Drawing for the job (mm, zero at the part's lowest x, y, z). A direction names the side the tool comes from. Give positions to 0.01 mm unless a question says otherwise; leave off trailing zeros. Order: outer loops, then holes, each group sorted by start corner. A loop starts at its lowest first (then second) coordinate and runs counter-clockwise, first axis right, second up. Notation, with made-up numbers: (70, 22.25) - (94, 22.25) arc R15 cw to (94, 47.25) - close; hole circle Ø6 at (35.25, 39.5). An arc over 180 degrees is marked (long way). Use a Markdown table: item, result. Add a question column.
(1) Flat gauge pins, fed straight in: pin 1 (10 mm diameter, centred on x = 56.5, z = 29, fed in from +Y); pin 2 (1.5 mm diameter, centred on x = 40, y = 25.5, fed in from -Z); pin 3 (1.1 mm diameter, centred on x = 49, y = 56, fed in from +Z); pin 4 (1 mm diameter, centred on x = 8, y = 47, fed in from +Z). Where does each tip first touch, or does it go through?
(2) Slice it at B-B (x = 39). Write the cut outline in (y, z).
(3) Mould opens along Y. For the marked faces 3, 4 and 5 say: +Y half, -Y half, draft (parallel to the pull), parting line (faces both ways), or undercut.
(4) Which spindle directions (+Z, -Z, +X, -X, +Y, -Y) get a long thin tool onto all of the face, cutting with end or side? Do the marked faces 1 and 2. Say none if no direction does.
(5) Wall check: line 1 (Y direction, x = 25.5, z = 32); line 2 (Z direction, x = 46.5, y = 16); line 3 (Y direction, x = 46, z = 11). Give the ranges that are in metal, low to high.
(6) Slice it at D-D (z = 17.5). Write the cut outline in (x, y).
(7) Slice it at A-A (z = 6). Write the cut outline in (x, y).
(8) Slice it at C-C (y = 31). Write the cut outline in (x, z), then the cut area to 3 significant figures.
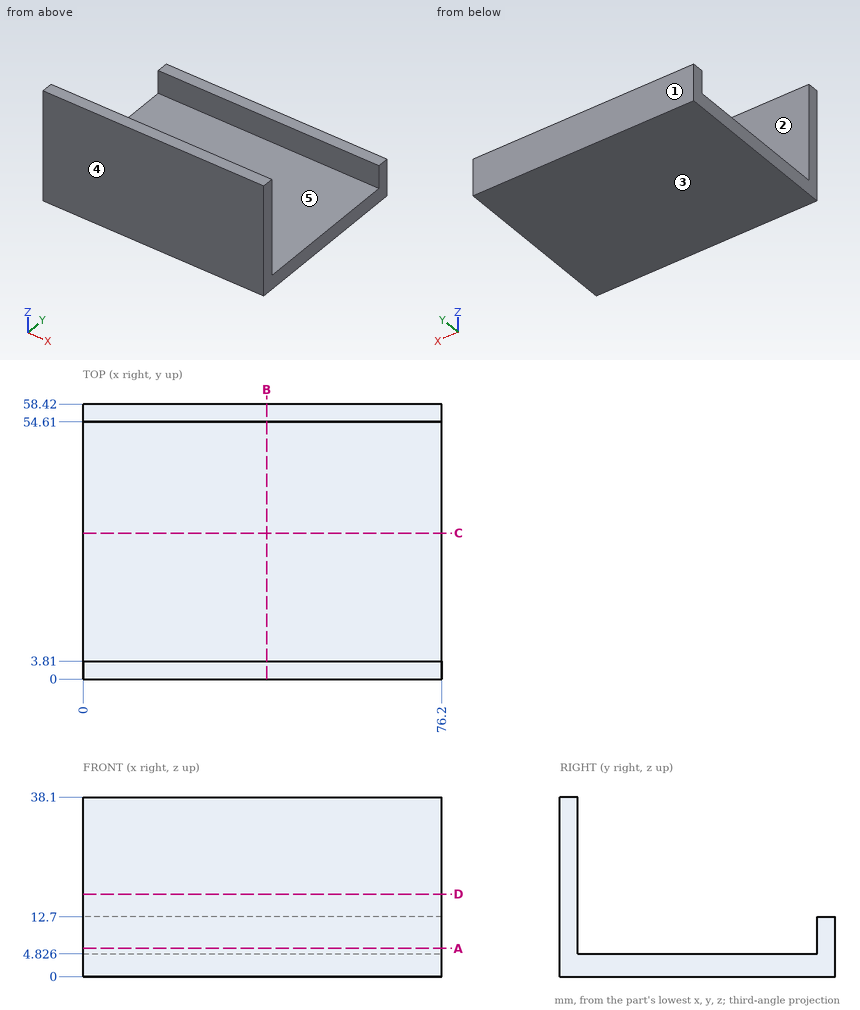
Solution:
| question | item | result |
|---|---|---|
| 1 | pin 1 | y = 3.81 |
| 1 | pin 2 | z = 0 |
| 1 | pin 3 | z = 12.7 |
| 1 | pin 4 | z = 4.83 |
| 2 | outline | (0, 0) - (58.42, 0) - (58.42, 12.7) - (54.61, 12.7) - (54.61, 4.83) - (3.81, 4.83) - (3.81, 38.1) - (0, 38.1) - close |
| 3 | face 3 | draft |
| 3 | face 4 | -Y half |
| 3 | face 5 | undercut |
| 4 | face 1 | +Z, -Z, +X, -X, +Y |
| 4 | face 2 | +Z, +X, -X |
| 5 | line 1 | 0 to 3.81 |
| 5 | line 2 | 0 to 4.83 |
| 5 | line 3 | 0 to 3.81, 54.61 to 58.42 |
| 6 | outline | (0, 0) - (76.2, 0) - (76.2, 3.81) - (0, 3.81) - close |
| 7 | outline | (0, 0) - (76.2, 0) - (76.2, 3.81) - (0, 3.81) - close; (0, 54.61) - (76.2, 54.61) - (76.2, 58.42) - (0, 58.42) - close |
| 8 | outline | (0, 0) - (76.2, 0) - (76.2, 4.83) - (0, 4.83) - close |
| 8 | area | 368 mm2 |
